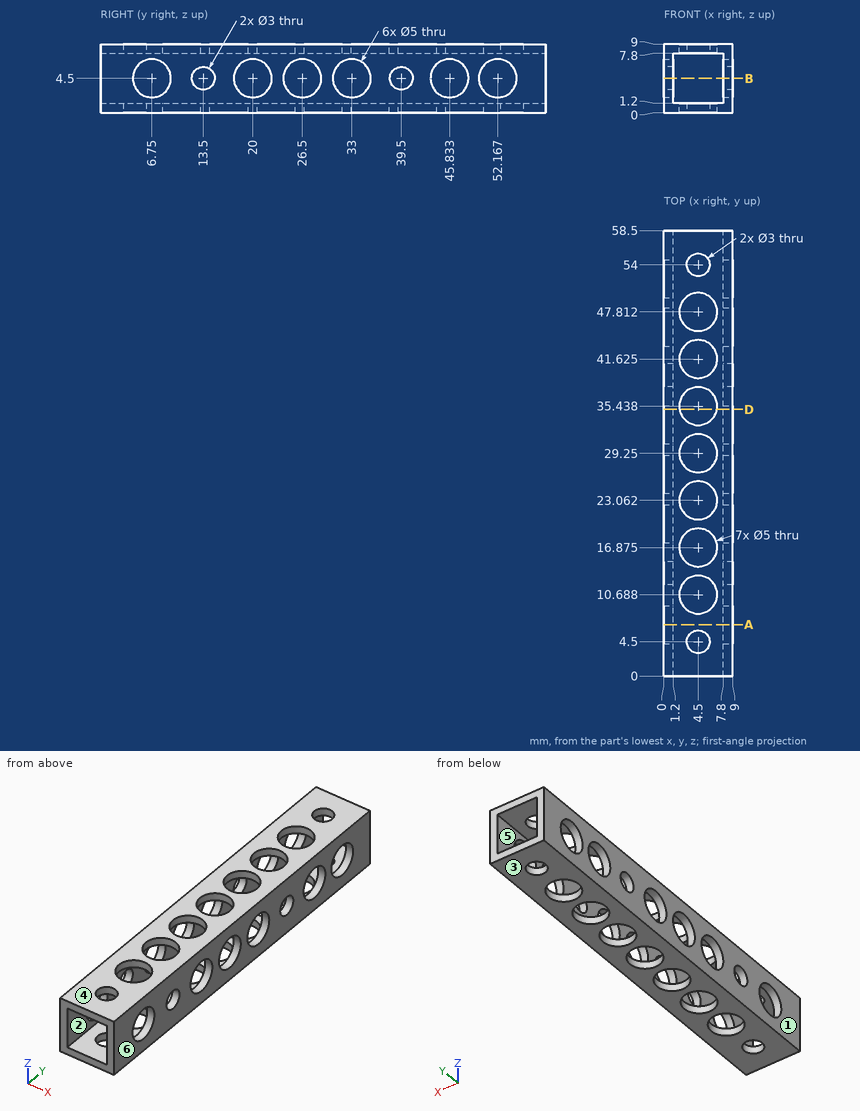
Job drawing, mm, ordinate dimensions from the low corner. One solid piece. A direction names the side the tool comes from. Give positions to 0.01 mm unless a question says otherwise; leave off trailing zeros. Write each loop counter-clockwise with the first axis right and the second up, starting at its lowest first coordinate (ties: lowest second). Pieces come first, ordered by that corner, then holes. Notation, with made-up numbers: (74, -21.5) -> (84, -21.5) arc R30 cw to (84, 2.5) -> close; hole circle Ø5 at (60.5, 53). An arc over 180 degrees is marked (long way). Return JSON: item names as keys, results as strings.
Item 1: Drill centre lines: probe 1 along X at (y, z) = (4, 7.25); probe 2 along X at (y, z) = (4.5, 0.6). Where is each one in solid material? Low to high.
Answer below:
{"probe 1": "x = 0 to 1.2, 7.8 to 9", "probe 2": "x = 0 to 3, 6 to 9"}
Item 2: Band-saw the part on B-B (z = 4.5). Give the number of separate pieces and of enclosed holes in the cut face.
Answer below:
{"separate pieces": "18", "enclosed holes": "0"}
Item 3: Tool access for the marked faces 1 and 2: list every direction of +Z, -Z, +X, -X, +Y, -Y with a clear straight run to the whole face (end or side of a thin tool).
Answer below:
{"face 1": "+Z, -Z, -X, +Y, -Y", "face 2": "+Y, -Y"}
Item 4: Two-plate mould, pull along Z, no slides. Class the marked faces 3, 4, 5 and 6: +Z half, -Z half, draft (parallel to the pull), parting line (faces both ways), or undercut.
Answer below:
{"face 3": "-Z half", "face 4": "+Z half", "face 5": "undercut", "face 6": "draft"}
Item 5: Band-saw the part on A-A (y = 6.75). List the corners of the cut face in (x, z).
Answer below:
{"outline": "(0, 0) -> (9, 0) -> (9, 2) -> (7.8, 2) -> (7.8, 1.2) -> (1.2, 1.2) -> (1.2, 2) -> (0, 2) -> close; (0, 7) -> (1.2, 7) -> (1.2, 7.8) -> (7.8, 7.8) -> (7.8, 7) -> (9, 7) -> (9, 9) -> (0, 9) -> close"}
Item 6: Band-saw the part on D-D (y = 35). List the corners of the cut face in (x, z).
Answer below:
{"outline": "(0, 0) -> (2.04, 0) -> (2.04, 1.2) -> (1.2, 1.2) -> (1.2, 3) -> (0, 3) -> close; (0, 6) -> (1.2, 6) -> (1.2, 7.8) -> (2.04, 7.8) -> (2.04, 9) -> (0, 9) -> close; (6.96, 0) -> (9, 0) -> (9, 3) -> (7.8, 3) -> (7.8, 1.2) -> (6.96, 1.2) -> close; (6.96, 7.8) -> (7.8, 7.8) -> (7.8, 6) -> (9, 6) -> (9, 9) -> (6.96, 9) -> close"}
